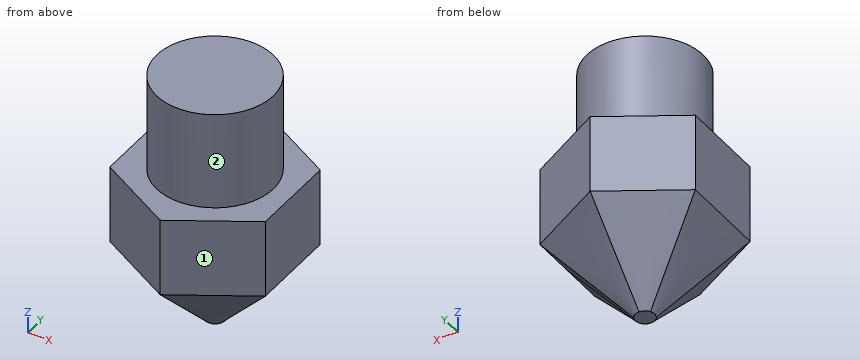
```python
from build123d import *

# Parameters (mm, degrees)
F0_R     = 3
F1_DEPTH = 5
F2_DEPTH = 4
F4_R     = 0.5


with BuildPart() as f1:
    # F0 (on Top) → F1 (new body)
    with BuildSketch(Plane.XY):
        Circle(F0_R)
    extrude(amount=F1_DEPTH)

    # F0 (on Top) → F2 (join)
    with BuildSketch(Plane.XY):
        Polygon((4, -2.309401), (4, 2.309401), (0, 4.618802), (-4, 2.309401), (-4, -2.309401), (0, -4.618802), align=None)
        Circle(F0_R, mode=Mode.SUBTRACT)
        Circle(F0_R)
    extrude(amount=-F2_DEPTH)

    # F2_face (on face) → F5 section 0
    with BuildSketch(Plane(origin=(0, 0, -4), x_dir=(1, 0, 0), z_dir=(0, 0, -1))):
        Polygon((4, -2.309401), (4, 2.309401), (0, 4.618802), (-4, 2.309401), (-4, -2.309401), (0, -4.618802), align=None)
    # F4 (on offset) → F5 section 1
    with BuildSketch(Plane.XY.offset(-8)):
        Circle(F4_R)
    loft()


solid = f1.part
```
Work out the finished part from the listing and answer in its coordinate system (mm). Face numbers are marked on the shaded views. A direction names the side the tool comes from. Round coordinates to 2 decimals unless told otherwise and drop trailing zeros. Loops run counter-clockwise (first coordinate to the right, second up) from the corner with the lowest first, then second, coordinate; pieces in that order, holes last. Notation, with made-up numbers: M 84,0 L 93,0 A11 cw 93,6 Z; hole C 23.5,3.5 d9. An arc over 180 degrees is marked long. One line per question, with ' | ' between items.
Q1. Consider line 1 along Y through (x, z) = (-2.25, 0.5); line 2 along Z through (x, y) = (0.25, -2); line 3 along Y through (x, z) = (-0.5, -1.5). Determine where each line is inside the solid, lowest interval first. Write a range as from..to.
Conclusion:
line 1: y = -1.98..1.98 | line 2: z = -6.42..5 | line 3: y = -4.33..4.33
Q2. A tool of negligible diameter and unlimited length cuts with its end or side. For the marked faces 1 and 2, from which of +Z, -Z, +X, -X, +Y, -Y can it reach the whole face along a straight path? Write none if from no direction.
Conclusion:
face 1: +Z, -Z, +X, -Y | face 2: +Z
Q3. Find section B-B, the plane z = 1. Give the vertices of the cut face in (x, y).
Conclusion:
outline: C 0,0 d6
Q4. Each of these flat-tipped pins is pushed along its axis until it touches: pin 1 Ø2 at (x, z) = (-2.5, 1.5) entering from +Y; pin 2 Ø1.5 at (x, z) = (-0.5, -3) entering from +Y; pin 3 Ø1 at (x, y) = (-2.5, -3) entering from -Z. Where does it stop, or does it pass through?
Conclusion:
pin 1: stops at y = 2.6 | pin 2: stops at y = 4.62 | pin 3: stops at z = -4.74
Q5. Find section A-A, the plane z = -1.75. Give the vertices of the cut face in (x, y).
Conclusion:
outline: M -4,-2.31 L 0,-4.62 L 4,-2.31 L 4,2.31 L 0,4.62 L -4,2.31 Z
